Could you check a few things on this model? Use its own coordinates, in mm. A direction names the side the tool comes from. Round coordinates to 2 decimals unless told otherwise and drop trailing zeros. Loops run counter-clockwise (first coordinate to the right, second up) from the corner with the lowest first, then second, coordinate; pieces in that order, holes last. Notation, with made-up numbers: M 12,-28 L 36,-28 A31 ccw 36,2 Z; hole C 60.25,65 d11. An arc over 180 degrees is marked long. Answer in a Markdown table with one row per item.
```python
from build123d import *

# Parameters (mm, degrees)
F0_W     = 10
F0_H     = 10
F0_R     = 6
F1_DEPTH = 10
F3_DEPTH = 3


with BuildPart() as f1:
    # F0 (on Top) → F1 (new body)
    with BuildSketch(Plane.XY):
        Polygon((10, 0), (0, 0), (-10, 0), (-10, -10), (-20, -10), (-20, -20), (-30, -20), (-30, -30), (-40, -30), (-40, -40), (-40, -50), (-30, -50), (-30, -60), (-40, -60), (-40, -70), (-30, -70), (-30, -80), (-20, -80), (-20, -70), (-25, -70), (-25, -60), (-20, -60), (-20, -50), (-10, -50), (-10, -60), (0, -60), (10, -60), (10, -50), (20, -50), (20, -60), (25, -60), (25, -70), (20, -70), (20, -80), (30, -80), (30, -70), (40, -70), (40, -60), (30, -60), (30, -50), (40, -50), (40, -40), (40, -30), (30, -30), (30, -20), (20, -20), (20, -10), (10, -10), align=None)
        with Locations((-15, -35)):
            Rectangle(F0_W, F0_H, mode=Mode.SUBTRACT)
        with Locations((15, -35)):
            Rectangle(F0_W, F0_H, mode=Mode.SUBTRACT)
        with Locations((0, -15)):
            Circle(F0_R, mode=Mode.SUBTRACT)
        with Locations((0, -15)):
            Circle(F0_R)
    extrude(amount=F1_DEPTH)

    # F2 (on Right) → F3 (cut, symmetric)
    with BuildSketch(Plane.YZ):
        Polygon((-30, 5), (-30, 0), (-24, 0), (-21.1132486541, 5), align=None)
    extrude(amount=F3_DEPTH, both=True, mode=Mode.SUBTRACT)


solid = f1.part
```
1) I want a section at A-A, the plane y = -39. Please give me the cut outline in (x, z), plus the area to 3 significant figures.
Computed:
| item | result |
|---|---|
| outline | M -40,0 L -20,0 L -20,10 L -40,10 Z; M -10,0 L 10,0 L 10,10 L -10,10 Z; M 20,0 L 40,0 L 40,10 L 20,10 Z |
| area | 600 mm² |
2) I want a section at C-C, the plane y = -72. Please give me the cut outline in (x, z), plus the area to 3 significant figures.
Computed:
| item | result |
|---|---|
| outline | M -30,0 L -20,0 L -20,10 L -30,10 Z; M 20,0 L 30,0 L 30,10 L 20,10 Z |
| area | 200 mm² |
3) If we mould it in two halves opening along Z, with no side actions, what happens to faces 4 (the face through (0, -25, 5)), 5 (the face through (10, -35, 5)), 6 (the face through (-1, -39, 0))? For each: released by +Z, released by -Z, zero draft, split by the parting line, or undercut.
Computed:
| item | result |
|---|---|
| face 4 | undercut |
| face 5 | zero draft |
| face 6 | released by -Z |
4) I need wall thicknesses on line 1 (X direction, y = -59.5, z = 3.5); line 2 (X direction, y = -39, z = 4.75); line 3 (Y direction, x = 35, z = 6.75). Which ranges of each line are inside material? Lowest first, please.
Computed:
| item | result |
|---|---|
| line 1 | x = -30 to -20, -10 to 10, 20 to 30 |
| line 2 | x = -40 to -20, -10 to 10, 20 to 40 |
| line 3 | y = -70 to -60, -50 to -30 |
5) I want a section at D-D, the plane z = 6.5. State how many separate pieces and enclosed holes the cut face has, plus the area to 3 significant figures.
Computed:
| item | result |
|---|---|
| separate pieces | 1 |
| enclosed holes | 2 |
| area | 3,500 mm² |
6) Will these pins go through, and if not, where does the flat tip stop? P1, Ø1, axis at x = 14.5, z = 9, coming from the -Y side; P2, Ø3, axis at x = 17, z = 7, coming from the +Y side; P3, Ø6, axis at y = -54, z = 6.5, coming from the -X side; P4, Ø3, axis at x = -28.5, y = -40, coming from the -Z side.
Computed:
| item | result |
|---|---|
| P1 | stops at y = -50 |
| P2 | stops at y = -10 |
| P3 | stops at x = -30 |
| P4 | stops at z = 0 |
7) I want a section at B-B, the plane x = 33.5. Please give me the cut outline in (y, z).
Computed:
| item | result |
|---|---|
| outline | M -70,0 L -60,0 L -60,10 L -70,10 Z; M -50,0 L -30,0 L -30,10 L -50,10 Z |
8) Which directions (+Z, -Z, +X, -X, +Y, -Y) give clear straight access to the entire face, cutting with the end or side of a thin tool? Please do faces 1 (the face through (-20, -15, 5)), 2 (the face through (22, -60, 5)), 3 (the face through (-30, -55, 5)).
Computed:
| item | result |
|---|---|
| face 1 | +Z, -Z, -X, +Y |
| face 2 | +Z, -Z |
| face 3 | +Z, -Z, -X |
